Design review of the part shown in the three views and the two pictorial views. Dimensions are in mm from the part's minimum x, y and z. A direction names the side the tool comes from. Coordinates: 2 decimals unless noted, no trailing zeros. Loops run counter-clockwise (first coordinate to the right, second up) from the corner with the lowest first, then second, coordinate; pieces in that order, holes last. Notation, with made-up numbers: (3, -29.75) -> (18, -29.75) arc R27 ccw to (18, 0.25) -> close; hole circle Ø7 at (-23.75, -28). An arc over 180 degrees is marked (long way). One line per item, written item: value.
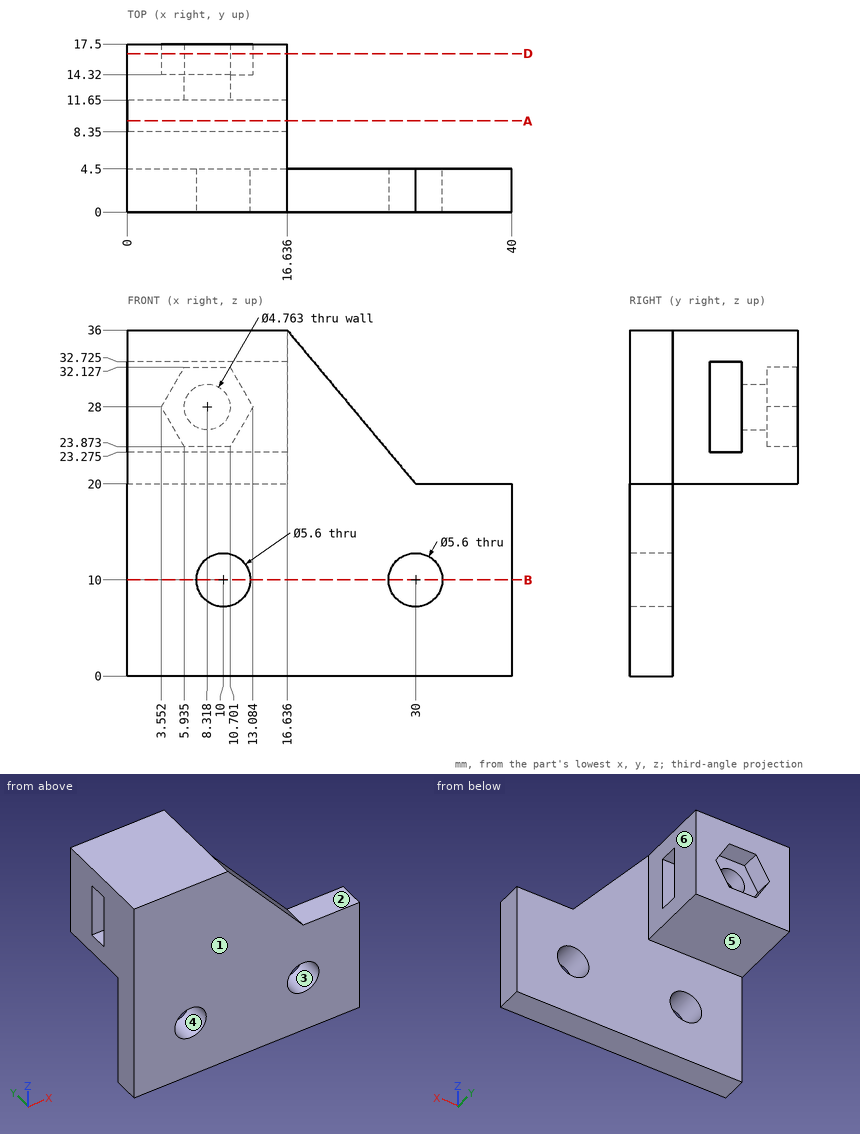
1. The part is to be moulded in two halves that separate along X. For the marked faces 3, 4, 5 and 6, say which applies: pulls with the +X half, pulls with the -X half, needs draft (parallel to the pull), parting line crosses it, or undercut.
Return value:
face 3: undercut
face 4: undercut
face 5: needs draft
face 6: pulls with the +X half
2. Take a section at D-D, the plane y = 16.5. Give the boundary of the cut face in (x, z) (1 decimal).
Return value:
outline: (0, 20) -> (16.6, 20) -> (16.6, 36) -> (0, 36) -> close; hole (3.6, 28) -> (5.9, 23.9) -> (10.7, 23.9) -> (13.1, 28) -> (10.7, 32.1) -> (5.9, 32.1) -> close
3. Take a section at B-B, the plane z = 10. Give the boundary of the cut face in (x, y), and give its area (3 significant figures).
Return value:
outline: (0, 0) -> (7.2, 0) -> (7.2, 4.5) -> (0, 4.5) -> close; (12.8, 0) -> (27.2, 0) -> (27.2, 4.5) -> (12.8, 4.5) -> close; (32.8, 0) -> (40, 0) -> (40, 4.5) -> (32.8, 4.5) -> close
area: 130 mm2
4. Take a section at A-A, the plane y = 9.5. Give the boundary of the cut face in (x, z) (1 decimal), and give its area (3 significant figures).
Return value:
outline: (0, 20) -> (16.6, 20) -> (16.6, 23.3) -> (0, 23.3) -> close; (0, 32.7) -> (16.6, 32.7) -> (16.6, 36) -> (0, 36) -> close
area: 109 mm2
5. Insertion check: pin 1 Ø9 at (x, z) = (10, 10) entering from -Y; pin 2 Ø3 at (x, y) = (30.5, 3) entering from +Z (1 decimal); pin 3 Ø1.7 at (x, y) = (12, 10.5) entering from -Z; pin 4 Ø8 at (x, z) = (29.5, 8) entering from +Y. Each pin has a flat end and moves straight along its axis. Give the tip position at first contact, or say it passes through.
Return value:
pin 1: stops at y = 0
pin 2: stops at z = 21.2
pin 3: stops at z = 20
pin 4: stops at y = 4.5
6. To check wall thickness, follow probe 1 along X at (y, z) = (2.85, 10); probe 2 along Z at (x, y) = (10, 2.4); probe 3 along Z at (x, y) = (7.5, 16.5). State the ranges of each line that lie inside material, in increasing order. Write a range as from..to.
Return value:
probe 1: x = 0..7.2, 12.8..27.2, 32.8..40
probe 2: z = 0..7.2, 12.8..36
probe 3: z = 20..23.87, 32.13..36
7. For the marked faces 1 and 2, list the 3-axis set-ups (+Z, -Z, +X, -X, +Y, -Y) from which the entire face can be reached by the end or side of a thin tool; tool diameter is ignored.
Return value:
face 1: +Z, -Z, +X, -X, -Y
face 2: +Z, +X, +Y, -Y
